Autodesk Inventor part; units mm, degrees
ref_plane "YZ Plane" through (0, 0, 0) normal (1, 0, 0) x (0, 1, 0)
ref_plane "XZ Plane" through (0, 0, 0) normal (0, 1, 0) x (-1, 0, 0)
ref_plane "XY Plane" through (0, 0, 0) normal (0, 0, 1) x (1, 0, 0)
sketch "Sketch1" plane through (0, 0, 0) normal (0, 1, 0) x (-1, 0, 0)
  line L0 (175, -115) -> (-175, -115)
  line L1 (-175, -115) -> (-175, 115)
  line L2 (-175, 115) -> (175, 115)
  line L3 (175, 115) -> (175, -115)
  line L4 (0, -115) -> (0, 115) construction
  line L5 (175, 0) -> (-175, 0) construction
  point P0 (0, 0)
  point P1 (0, 0)
  dimension "d0" = 350
  dimension "d1" = 230
extrude "Extrusion1" add sketch "Sketch1" along normal blind 3
sketch "Sketch2" plane through (0, 0, 0) normal (0, -1, 0) x (1, 0, 0)
  line L0 (175, -115) -> (-175, -115) construction
  line L1 (0, -115) -> (0, 115) construction
  line L2 (-175, 115) -> (175, 115) construction
  line L3 (130, -40) -> (110, -40)
  line L4 (110, -40) -> (110, 40)
  line L5 (110, 40) -> (130, 40)
  line L6 (130, 40) -> (130, -40)
  line L7 (130, 0) -> (110, 0) construction
  line L8 (0, 0) -> (175, 0) construction
  line L9 (175, 115) -> (175, -115) construction
  line L10 (-130, -40) -> (-110, -40)
  line L11 (-110, -40) -> (-110, 40)
  line L12 (-110, 40) -> (-130, 40)
  line L13 (-130, 40) -> (-130, -40)
  dimension "d4" = 20
  dimension "d5" = 80
  dimension "d6" = 220
extrude "Extrusion2" add sketch "Sketch2" along normal blind 10
sketch "Sketch3" plane through (0, -10, 0) normal (0, -1, 0) x (1, 0, 0)
  line L0 (175, 115) -> (-175, 115) construction
  line L1 (0, 115) -> (0, -115) construction
  line L2 (175, -115) -> (-175, -115) construction
  line L3 (0, 0) -> (-175, 0) construction
  line L4 (-175, 115) -> (-175, -115) construction
  line L5 (-110, 40) -> (-130, 40) construction
  line L6 (-120, 40) -> (-120, -40) construction
  line L7 (-130, -40) -> (-110, -40) construction
  circle A0 centre (-120, 25) radius 2.75
  circle A1 centre (-120, -25) radius 2.75
  circle A2 centre (120, 25) radius 2.75
  circle A3 centre (120, -25) radius 2.75
  dimension "d9" = 5.5
  dimension "d10" = 15
extrude "Extrusion3" cut sketch "Sketch3" against normal up to next
sketch "Sketch4" plane through (0, 0, 0) normal (0, -1, 0) x (1, 0, 0)
  line L0 (110, 40) -> (110, -40) construction
  line L1 (110, 0) -> (-110, 0) construction
  line L2 (-110, -40) -> (-110, 40) construction
  line L3 (110, 15) -> (-110, 15)
  line L4 (-110, 15) -> (-110, 20)
  line L5 (-110, 20) -> (110, 20)
  line L6 (110, 20) -> (110, 15)
  line L7 (110, -15) -> (-110, -15)
  line L8 (-110, -15) -> (-110, -20)
  line L9 (-110, -20) -> (110, -20)
  line L10 (110, -20) -> (110, -15)
  point P0 (0, 0)
  dimension "d13" = 5
  dimension "d14" = 30
extrude "Extrusion4" add sketch "Sketch4" along normal blind 5
fillet "Fillet1" radius 10 6 edges at (120, 0, 40) (130, 0, 0) (120, 0, -40) (-120, 0, 40) (-130, 0, 0) (-120, 0, -40)
fillet "Fillet2" radius 5 4 edges at (0, 0, 20) (0, 0, -15) (0, 0, 15) (0, 0, -20)
sketch "Sketch5" plane through (0, 3, 0) normal (0, 1, 0) x (1, 0, 0)
  line L0 (-175, -115) -> (-175, 115) construction
  line L1 (-175, 0) -> (175, 0) construction
  line L2 (175, -115) -> (175, 115) construction
  line L3 (175, -115) -> (-175, -115) construction
  line L4 (0, -115) -> (0, 115) construction
  line L5 (-175, 115) -> (175, 115) construction
  circle A0 centre (-120, 25) radius 2.75
  circle A1 centre (-120, 25) radius 4.5
  circle A2 centre (-120, -25) radius 4.5
  circle A3 centre (120, 25) radius 4.5
  circle A4 centre (120, -25) radius 4.5
  point P0 (0, 0)
  dimension "d19" = 9
extrude "Extrusion5" cut sketch "Sketch5" against normal blind 6
sketch "Sketch6" plane through (0, 3, 0) normal (0, 1, 0) x (1, 0, 0)
  line L0 (175, 115) -> (-175, 115) construction
  line L1 (0, 115) -> (0, -115) construction
  line L2 (175, -115) -> (-175, -115) construction
  line L3 (-175, 115) -> (-175, -115) construction
  line L4 (-175, 0) -> (175, 0) construction
  line L5 (175, -115) -> (175, 115) construction
  circle A0 centre (-179, 119) radius 6
  line L6 (-175, 115) -> (-179, 115) construction
  line L7 (-179, 115) -> (-179, 119) construction
  line L8 (-179, 119) -> (-175, 119) construction
  line L9 (-175, 119) -> (-175, 115) construction
  line L10 (-155, 115) -> (-175.4528, 123.8392)
  line L11 (-175, 95) -> (-183.0203, 114.5461)
  line L12 (-175, 95) -> (-175, 115)
  line L13 (-155, 115) -> (-175, 115)
  circle A1 centre (-179, -119) radius 6
  line L14 (-155, -115) -> (-175.4528, -123.8392)
  line L15 (-175, -95) -> (-183.0203, -114.5461)
  line L16 (-175, -95) -> (-175, -115)
  line L17 (-155, -115) -> (-175, -115)
  circle A2 centre (179, 119) radius 6
  line L18 (155, 115) -> (175.4528, 123.8392)
  line L19 (175, 95) -> (183.0203, 114.5461)
  line L20 (175, 95) -> (175, 115)
  line L21 (155, 115) -> (175, 115)
  line L22 (175, -95) -> (183.0203, -114.5461)
  circle A3 centre (179, -119) radius 6
  line L23 (155, -115) -> (175.4528, -123.8392)
  line L24 (155, -115) -> (175, -115)
  line L25 (175, -95) -> (175, -115)
  circle A4 centre (179, -119) radius 2.75
  circle A5 centre (179, 119) radius 2.75
  circle A6 centre (-179, -119) radius 2.75
  circle A7 centre (-179, 119) radius 2.75
  point P0 (0, 0)
  dimension "d22" = 12
  dimension "d23" = 4
  dimension "d24" = 4
  dimension "d25" = 20
  dimension "d26" = 20
  dimension "d30" = 5.5
extrude "Extrusion6" add sketch "Sketch6" against normal blind 3 contours A0 L13 L12 | A0 L10 L13 | A0 L12 L11 | A1 L16 L17 | L15 L16 A1 | A1 L17 L14 | A2 L20 L21 | A2 L21 L18 | L19 L20 A2 | L22 A3 L25 | A3 L24 L25 | A3 L23 L24 picked at (-175.087, 116.3056) picked at (-175.087, -116.3056) picked at (175.0917, 116.2969) picked at (175.0917, -116.2969)
properties part number "vna_mount"
For this review, take the finished solid that the model builds, in its own axes (mm). A direction names the side the tool comes from. Give positions to 0.01 mm unless a question says otherwise; leave off trailing zeros. Order: outer loops, then holes, each group sorted by start corner. A loop starts at its lowest first (then second) coordinate and runs counter-clockwise, first axis right, second up.
1) Take a section at D-D (z = -75.5). Give the boundary of the cut face in (x, y), then the cut area to 3 significant figures.
2) For faces 1 (the face through (115.504, 0.042, -25.198)), 2 (the face through (-110, -5, -1)), 3 (the face through (-165.083, 1.521, 119.358)), list the 3-axis set-ups (+Z, -Z, +X, -X, +Y, -Y) from which the entire face can be reached by the end or side of a thin tool; tool diameter is ignored.
3) Wall thickness on line 1 (X direction, y = 0.2, z = 25); line 2 (Z direction, x = -120, y = 0.75); line 3 (Z direction, x = -179, y = 2.15): over which ranges is each line inside the solid? List them lowest first.
4) Take a section at B-B (y = -7.25). Give the boundary of the cut face in (x, z), then the cut area to 3 significant figures.
5) Insertion check: pin 1 (2.5 mm diameter, centred on x = 25.5, y = 2, fed in from +Z); pin 2 (3 mm diameter, centred on y = -6.5, z = -4, fed in from +X); pin 3 (6.5 mm diameter, centred on x = -179, z = -119, fed in from -Y); pin 4 (14.5 mm diameter, centred on x = 120, z = 25, fed in from +Y). Each pin has a flat end and moves straight along its axis. Give the tip position at first contact, or say it passes through.
6) The part is to be moulded in two halves that separate along X. For faces 4 (the face through (178.954, 1.521, 104.636)), 5 (the face through (165.083, 1.521, 119.358)), 6 (the face through (-121.46, -2.85, -43.01)), say which applies: released by +X, released by -X, zero draft, split by the parting line, or undercut.
Derived:
1. outline: (-175, 0) - (175, 0) - (175, 3) - (-175, 3) - close
1. area: 1,050 mm2
2. face 1: +Y
2. face 2: -Y
2. face 3: +Z, +Y, -Y
3. line 1: x = -175 to -124.5, -115.5 to 115.5, 124.5 to 175
3. line 2: z = -115 to -29.5, -20.5 to 20.5, 29.5 to 115
3. line 3: z = -125 to -121.75, -116.25 to -104.75, 104.75 to 116.25, 121.75 to 125
4. outline: (-130.39, -40.39) - (-110, -40.39) - (-110, 40.39) - (-130.39, 40.39) - close; (110, -40.39) - (130.39, -40.39) - (130.39, 40.39) - (110, 40.39) - close; hole circle Ø5.5 at (-120, -25); hole circle Ø5.5 at (-120, 25); hole circle Ø5.5 at (120, -25); hole circle Ø5.5 at (120, 25)
4. area: 3,200 mm2
5. pin 1: stops at z = 115
5. pin 2: stops at x = 131.34
5. pin 3: stops at y = 0
5. pin 4: stops at y = 3
6. face 4: released by +X
6. face 5: undercut
6. face 6: zero draft
